Check sheet for the modelled part. Datum: model origin and axes. Units: mm. A direction names the side the tool comes from. Round coordinates to 2 decimals unless told otherwise and drop trailing zeros. Order: outer loops, then holes, each group sorted by start corner. A loop starts at its lowest first (then second) coordinate and runs counter-clockwise, first axis right, second up. Notation, with made-up numbers: (40, 54) -> (79, 54) arc R24 ccw to (79, 71) -> close; hole circle Ø3 at (77, 82). An arc over 180 degrees is marked (long way). Use CSV: the item, a comma, the result in double quotes.
```python
from build123d import *

# Parameters (mm, degrees)
BOSS_EXTRUDE1_DEPTH = 3.5
SKETCH2_R           = 13.5
BOSS_EXTRUDE2_DEPTH = 5
SKETCH3_R           = 6
BOSS_EXTRUDE3_DEPTH = 4
SKETCH4_R           = 4
CUT_EXTRUDE1_DEPTH  = 31.24070105
SKETCH5_R           = 2.4
CUT_EXTRUDE2_DEPTH  = 29.969811874


with BuildPart() as part:
    # Sketch1 → Boss-Extrude1 (new body)
    with BuildSketch(Plane(origin=(0, 0, 0), x_dir=(1, 0, 0), z_dir=(0, 1, 0))):
        with BuildLine():
            Line((-20.657112668, 5.059334436), (-9.221211054, 9.935178986))
            ThreePointArc((-9.221211054, 9.935178986), (-9.078911878, 10.009890435), (-8.950419333, 10.106433286))
            ThreePointArc((-8.950419333, 10.106433286), (0, 13.5), (8.950419333, 10.106433286))
            ThreePointArc((8.950419333, 10.106433286), (9.078911878, 10.009890435), (9.221211054, 9.935178986))
            Line((9.221211054, 9.935178986), (20.657112668, 5.059334436))
            ThreePointArc((20.657112668, 5.059334436), (24, 0), (20.657112668, -5.059334436))
            Line((20.657112668, -5.059334436), (9.221211054, -9.935178986))
            ThreePointArc((9.221211054, -9.935178986), (9.078911878, -10.009890435), (8.950419333, -10.106433286))
            ThreePointArc((8.950419333, -10.106433286), (0, -13.5), (-8.950419333, -10.106433286))
            ThreePointArc((-8.950419333, -10.106433286), (-9.078911878, -10.009890435), (-9.221211054, -9.935178986))
            Line((-9.221211054, -9.935178986), (-20.657112668, -5.059334436))
            ThreePointArc((-20.657112668, -5.059334436), (-24, 0), (-20.657112668, 5.059334436))
        make_face()
    extrude(amount=BOSS_EXTRUDE1_DEPTH)

    # Sketch2 → Boss-Extrude2 (add)
    with BuildSketch(Plane(origin=(0, 3.5, 0), x_dir=(1, 0, 0), z_dir=(0, 1, 0))):
        with Locations(Location((0, 0, 0), (0, 0, 131.528615852))):
            Circle(SKETCH2_R)
    extrude(amount=BOSS_EXTRUDE2_DEPTH)

    # Sketch3 → Boss-Extrude3 (add)
    with BuildSketch(Plane(origin=(0, 8.5, 0), x_dir=(1, 0, 0), z_dir=(0, 1, 0))):
        with Locations(Location((0, 0, 0), (0, 0, 270))):
            Circle(SKETCH3_R)
    extrude(amount=BOSS_EXTRUDE3_DEPTH)

    # Sketch4 → Cut-Extrude1 (cut, through all)
    with BuildSketch(Plane(origin=(0, 12.5, 0), x_dir=(1, 0, 0), z_dir=(0, 1, 0))):
        with Locations(Location((0, 0, 0), (0, 0, 270))):
            Circle(SKETCH4_R)
    extrude(amount=-CUT_EXTRUDE1_DEPTH, mode=Mode.SUBTRACT)

    # Sketch5 → Cut-Extrude2 (cut, through all)
    with BuildSketch(Plane(origin=(0, 3.5, 0), x_dir=(1, 0, 0), z_dir=(0, 1, 0))):
        with Locations(Location((-18.5, 0, 0), (0, 0, 270))):
            Circle(SKETCH5_R)
        with Locations(Location((18.5, 0, 0), (0, 0, 270))):
            Circle(SKETCH5_R)
    extrude(amount=-CUT_EXTRUDE2_DEPTH, mode=Mode.SUBTRACT)


solid = part.part
```
Q1. Access from +Z, -Z, +X, -X, +Y, -Y to the whole of each face (thin tool, end or side, straight path). Record for faces 5 (the face through (24, 2, 0)), 6 (the face through (2, 8.5, -6)).
Result sheet:
face 5,"+X, +Y, -Y"
face 6,"+Y"
Q2. Scan lines: L1, parallel to X at y = 10, z = 0; L2, parallel to X at y = 1.75, z = -1.5; L3, parallel to Y at x = 20, z = -5.25. Record each from-to range of solid material in increasing order.
Result sheet:
L1,"x = -6 to -4, 4 to 6"
L2,"x = -23.79 to -20.37, -16.63 to -3.71, 3.71 to 16.63, 20.37 to 23.79"
L3,"y = 0 to 3.5"
Q3. Sectioned sample at B-B, the plane y = 1. Enter the section's corners in (x, z).
Result sheet:
outline,"(-20.66, -5.06) -> (-9.22, -9.94) arc R1 cw to (-8.95, -10.11) arc R13.5 ccw to (8.95, -10.11) arc R1 cw to (9.22, -9.94) -> (20.66, -5.06) arc R5.5 ccw to (20.66, 5.06) -> (9.22, 9.94) arc R1 cw to (8.95, 10.11) arc R13.5 ccw to (-8.95, 10.11) arc R1 cw to (-9.22, 9.94) -> (-20.66, 5.06) arc R5.5 ccw to start; hole circle Ø4.8 at (-18.5, 0); hole circle Ø8 at (0, 0); hole circle Ø4.8 at (18.5, 0)"
Q4. Sectioned sample at A-A, the plane z = 0. Enter the section's corners in (x, y), then the cut area to 3 significant figures.
Result sheet:
outline,"(-24, 0) -> (-20.9, 0) -> (-20.9, 3.5) -> (-24, 3.5) -> close; (-16.1, 0) -> (-4, 0) -> (-4, 12.5) -> (-6, 12.5) -> (-6, 8.5) -> (-13.5, 8.5) -> (-13.5, 3.5) -> (-16.1, 3.5) -> close; (4, 0) -> (16.1, 0) -> (16.1, 3.5) -> (13.5, 3.5) -> (13.5, 8.5) -> (6, 8.5) -> (6, 12.5) -> (4, 12.5) -> close; (20.9, 0) -> (24, 0) -> (24, 3.5) -> (20.9, 3.5) -> close"
area,"217 mm^2"
Q5. Mould release check, pull along Z, two halves, no side actions. Record for faces 1 (the face through (14.86, 1.73, -7.53)), 2 (the face through (1.802, 10.472, 5.723)), 3 (the face through (-3.905, 6.338, -0.867)), 4 (the face through (16.157, 1.774, -0.52)): pulls with the +Z half, pulls with the -Z half, needs draft (parallel to the pull), parting line crosses it, or undercut.
Result sheet:
face 1,"pulls with the -Z half"
face 2,"parting line crosses it"
face 3,"undercut"
face 4,"undercut"
Q6. Sectioned sample at D-D, the plane y = 4.5. Enter the section's corners in (x, z), then the cut area to 3 significant figures.
Result sheet:
outline,"circle Ø27 at (0, 0); hole circle Ø8 at (0, 0)"
area,"522 mm^2"
Q7. Go/stop test with flat-tipped pins: pin 1 (1 mm diameter, centred on y = 3, z = 10, fed in from +X); pin 2 (4 mm diameter, centred on y = 6, z = -9.5, fed in from +X) (3 decimals); pin 3 (6 mm diameter, centred on y = 10.5, z = -8.5, fed in from +X). Record where each tip stops, or that it passes through.
Result sheet:
pin 1,"stops at x = 10.24"
pin 2,"stops at x = 11.225"
pin 3,"stops at x = 11.96"
Q8. Sectioned sample at C-C, the plane x = 0. Enter the section's corners in (y, z).
Result sheet:
outline,"(0, -13.5) -> (8.5, -13.5) -> (8.5, -6) -> (12.5, -6) -> (12.5, -4) -> (0, -4) -> close; (0, 4) -> (12.5, 4) -> (12.5, 6) -> (8.5, 6) -> (8.5, 13.5) -> (0, 13.5) -> close"
